Work out the finished part from the listing and answer in its coordinate system (mm). A direction names the side the tool comes from. Round coordinates to 2 decimals unless told otherwise and drop trailing zeros. Write each loop counter-clockwise with the first axis right and the second up, starting at its lowest first coordinate (ties: lowest second). Pieces come first, ordered by that corner, then holes. Notation, with made-up numbers: M 48.5,75 L 95.5,75 A14 ccw 95.5,82 Z; hole C -26.5,21.5 d5. An arc over 180 degrees is marked long. One line per item, written item: value. Start each with the question number.
Q1. The mould has two halves that part along X. Classify faces 5 (the flat face through (2, -1, 9)), 6 (the flat face through (-8, -5, 8)), 7 (the flat face through (6.959, -4.972, 9.214)): released by +X, released by -X, zero draft, split by the parting line, or undercut.
Q2. Find section A-A (y = -5.5). Write down the section's boundary in (x, z).
Q3. Find section B-B (x = 0). Write down the section's boundary in (y, z), and give its area (3 significant figures).
Q4. Find section C-C (y = -3.75). Write down the section's boundary in (x, z), and give its area (3 significant figures).
Q5. Consider probe 1 along Z at (x, y) = (0, -5.5); probe 2 along X at (y, z) = (-1.75, 4.5); probe 3 along Y at (x, z) = (6, 8.25). Determine where each line is inside the solid, lowest interval first.
Q6. Given pin 1 Ø1.7 at (x, z) = (-9, 4.5) entering from -Y; pin 2 Ø1.5 at (x, z) = (-3, -10.5) entering from -Y; pin 3 Ø0.9 at (y, z) = (-5, -10.5) entering from -X; pin 4 Ø0.6 at (y, z) = (-4, -10.5) entering from +X, each flat-ended and moving along its own axis, determine where each tip first touches the part or whether it passes through.
Q7. Find section D-D (z = 3). Count the separate pieces of the cut face and the enclosed holes in it, and give its area (3 significant figures).
Q8. A tool of negligible diameter and unlimited length cuts with its end or side. For faces 1 (the flat face through (4.5, -5, -11)), 2 (the flat face through (-8.837, -5.986, 7.411)), 3 (the flat face through (11, -5, 3)), 4 (the flat face through (-2, -1.7, -6.1)), from which of +Z, -Z, +X, -X, +Y, -Y can it reach the whole face along a straight path? Write none if from no direction.
from build123d import *

# Parameters (mm, degrees)
BOSS_EXTRUDE3_DEPTH = 7
BOSS_EXTRUDE4_DEPTH = 1
BOSS_EXTRUDE5_DEPTH = 7
BOSS_EXTRUDE6_DEPTH = 3
BOSS_EXTRUDE7_START = -5
BOSS_EXTRUDE7_DEPTH = 2
FILLET1_R           = 4


with BuildPart() as part:
    # Sketch1 → Boss-Extrude3 (new body)
    with BuildSketch(Plane(origin=(0, 0, 0), x_dir=(1, 0, 0), z_dir=(0, 1, 0))):
        with BuildLine():
            Line((2, 4.582575695), (2, 3.422298687))
            ThreePointArc((2, 3.422298687), (0, -3.96385271), (-2, 3.422298687))
            Line((-2, 3.422298687), (-2, 4.582575695))
            ThreePointArc((-2, 4.582575695), (0, -5), (2, 4.582575695))
        make_face()
    extrude(amount=-BOSS_EXTRUDE3_DEPTH)

    # Sketch1<6> → Boss-Extrude4 (add)
    with BuildSketch(Plane(origin=(0, 0, 0), x_dir=(1, 0, 0), z_dir=(0, 1, 0))):
        with BuildLine():
            Line((2, 10.816653826), (2, 4.582575695))
            ThreePointArc((2, 4.582575695), (0, -5), (-2, 4.582575695))
            Line((-2, 4.582575695), (-2, 10.816653826))
            ThreePointArc((-2, 10.816653826), (0, -11), (2, 10.816653826))
        make_face()
    extrude(amount=-BOSS_EXTRUDE4_DEPTH)

    # Sketch1<7> → Boss-Extrude5 (add)
    with BuildSketch(Plane(origin=(0, 0, 0), x_dir=(1, 0, 0), z_dir=(0, 1, 0))):
        with BuildLine():
            ThreePointArc((-7.460787851, -9.503640297), (0, -12.082323214), (7.460787851, -9.503640297))
            Line((7.460787851, -9.503640297), (6.442669325, -8.915829292))
            ThreePointArc((6.442669325, -8.915829292), (0, -11), (-6.442669325, -8.915829292))
            Line((-6.442669325, -8.915829292), (-7.460787851, -9.503640297))
        make_face()
        with BuildLine():
            Line((10.942669325, -1.121600658), (11.960787851, -1.709411663))
            ThreePointArc((11.960787851, -1.709411663), (12.051901073, -0.856863332), (12.082323214, 0))
            ThreePointArc((12.082323214, 0), (10.008820827, 6.768015949), (4.5, 11.21305196))
            Line((4.5, 11.21305196), (4.5, 10.03742995))
            ThreePointArc((4.5, 10.03742995), (9.233092656, 5.979130372), (11, 0))
            ThreePointArc((11, 0), (10.985657982, -0.561532466), (10.942669325, -1.121600658))
        make_face()
        with BuildLine():
            ThreePointArc((-4.5, 11.21305196), (-10.46359884, 6.041161607), (-11.960787851, -1.709411663))
            Line((-11.960787851, -1.709411663), (-10.942669325, -1.121600658))
            ThreePointArc((-10.942669325, -1.121600658), (-9.526279442, 5.5), (-4.5, 10.03742995))
            Line((-4.5, 10.03742995), (-4.5, 11.21305196))
        make_face()
    extrude(amount=-BOSS_EXTRUDE5_DEPTH)

    # Sketch1<8> → Boss-Extrude6 (add)
    with BuildSketch(Plane(origin=(0, 0, 0), x_dir=(1, 0, 0), z_dir=(0, 1, 0))):
        with BuildLine():
            Line((11.960787851, -1.709411663), (10.942669325, -1.121600658))
            ThreePointArc((10.942669325, -1.121600658), (9.526279442, -5.5), (6.442669325, -8.915829292))
            Line((6.442669325, -8.915829292), (7.460787851, -9.503640297))
            ThreePointArc((7.460787851, -9.503640297), (10.46359884, -6.041161607), (11.960787851, -1.709411663))
        make_face()
        with BuildLine():
            Line((4.5, 10.03742995), (4.5, 11.21305196))
            ThreePointArc((4.5, 11.21305196), (3.268930764, 11.631707781), (2, 11.915642419))
            Line((2, 11.915642419), (2, 10.816653826))
            ThreePointArc((2, 10.816653826), (3.273270148, 10.501699983), (4.5, 10.03742995))
        make_face()
        with BuildLine():
            Line((-7.460787851, -9.503640297), (-6.442669325, -8.915829292))
            ThreePointArc((-6.442669325, -8.915829292), (-9.526279442, -5.5), (-10.942669325, -1.121600658))
            Line((-10.942669325, -1.121600658), (-11.960787851, -1.709411663))
            ThreePointArc((-11.960787851, -1.709411663), (-10.46359884, -6.041161607), (-7.460787851, -9.503640297))
        make_face()
        with BuildLine():
            Line((-2, 10.816653826), (-2, 11.915642419))
            ThreePointArc((-2, 11.915642419), (-3.268930764, 11.631707781), (-4.5, 11.21305196))
            Line((-4.5, 11.21305196), (-4.5, 10.03742995))
            ThreePointArc((-4.5, 10.03742995), (-3.273270148, 10.501699983), (-2, 10.816653826))
        make_face()
    extrude(amount=-BOSS_EXTRUDE6_DEPTH)

    # Sketch1<9> → Boss-Extrude7 (add)
    with BuildSketch(Plane(origin=(0, 0, 0), x_dir=(1, 0, 0), z_dir=(0, 1, 0)).offset(BOSS_EXTRUDE7_START)):
        with BuildLine():
            ThreePointArc((-9.319249037, -7.689872017), (-8.438889046, -8.646830975), (-7.460787851, -9.503640297))
            Line((-7.460787851, -9.503640297), (-6.442669325, -8.915829292))
            ThreePointArc((-6.442669325, -8.915829292), (-7.458103894, -8.085585093), (-8.367496998, -7.140377721))
            Line((-8.367496998, -7.140377721), (-9.319249037, -7.689872017))
        make_face()
        with BuildLine():
            ThreePointArc((11.319249037, -4.225770402), (11.70781981, -2.984876806), (11.960787851, -1.709411663))
            Line((11.960787851, -1.709411663), (10.942669325, -1.121600658))
            ThreePointArc((10.942669325, -1.121600658), (10.731374042, -2.41611489), (10.367496998, -3.676276106))
            Line((10.367496998, -3.676276106), (11.319249037, -4.225770402))
        make_face()
        with BuildLine():
            Line((-2, 10.816653826), (-2, 11.915642419))
            ThreePointArc((-2, 11.915642419), (-3.268930764, 11.631707781), (-4.5, 11.21305196))
            Line((-4.5, 11.21305196), (-4.5, 10.03742995))
            ThreePointArc((-4.5, 10.03742995), (-3.273270148, 10.501699983), (-2, 10.816653826))
        make_face()
    extrude(amount=-BOSS_EXTRUDE7_DEPTH)

    # Fillet1
    fillet1_edges = [part.edges().sort_by_distance(p)[0] for p in [
        (0, -1, 5),
    ]]
    fillet(fillet1_edges, radius=FILLET1_R)


solid = part.part
The answers:
1. face 5: undercut
1. face 6: zero draft
1. face 7: released by +X
2. outline: M -11.96,1.71 A12.08 ccw -2,-11.92 L -2,-10.82 A11 cw -10.94,1.12 Z; M -9.32,7.69 L -8.37,7.14 A11 cw 6.44,8.92 L 7.46,9.5 A12.08 ccw Z; M -2,-4.58 L -2,-3.42 A3.96 cw long 2,-3.42 L 2,-4.58 A5 ccw long Z; M 4.5,-11.21 A12.08 ccw 11.32,4.23 L 10.37,3.68 A11 cw 4.5,-10.04 Z
3. outline: M -7,3.96 L 0,3.96 L 0,12.08 L -7,12.08 L -7,11 L -1,11 L -1,9 A4 cw -5,5 L -7,5 Z
3. area: 24.3 mm2
4. outline: M -11.96,1.71 A12.08 ccw -4.5,-11.21 L -4.5,-10.04 A11 cw -10.94,1.12 Z; M -7.46,9.5 L -6.44,8.92 A11 cw 6.44,8.92 L 7.46,9.5 A12.08 ccw Z; M -2,-4.8 L -2,-3.42 A3.96 cw long 2,-3.42 L 2,-4.8 A5.2 ccw long Z; M 4.5,-11.21 A12.08 ccw 11.96,1.71 L 10.94,1.12 A11 cw 4.5,-10.04 Z
4. area: 78.9 mm2
5. probe 1: 3.96 to 5, 11 to 12.08
5. probe 2: -11.21 to -10.04, -4.92 to 4.92, 10.04 to 11.21
5. probe 3: -1 to 0
6. pin 1: y = -1
6. pin 2: y = -7
6. pin 3: x = -6.71
6. pin 4: x = 6.48
7. separate pieces: 3
7. enclosed holes: 0
7. area: 49.9 mm2
8. face 1: -Z, -Y
8. face 2: -X, -Y
8. face 3: +Z
8. face 4: -Z, +Y, -Y
